```python
from build123d import *

# Parameters (mm, degrees)
BOSS_EXTRUDE1_DEPTH      = 5
BOSS_EXTRUDE1_DEPTH_BACK = 5
BODY_MOVE_COPY1_ANGLE    = 90
CUT_EXTRUDE2_DEPTH       = 708.325596879
CUT_EXTRUDE2_DEPTH_BACK  = 708.325596879
CUT_EXTRUDE3_DEPTH       = 30.3


with BuildPart() as part:
    # Sketch1 → Boss-Extrude1 (new, two sides: drawn at the far end of the back side and taken through both)
    with BuildSketch(Plane(origin=(164.5, 164.5, 0), x_dir=(-0.7071067811865478, 0.7071067811865475, 0), z_dir=(-0.7071067811865475, -0.7071067811865478, 0)).offset(-BOSS_EXTRUDE1_DEPTH_BACK)):
        Polygon((182.63813101, -115), (282.63813101, -115), (692.914393031, 0), (692.914393031, 10), (-227.63813101, 10), (-227.63813101, 0), align=None)
    extrude(amount=BOSS_EXTRUDE1_DEPTH + BOSS_EXTRUDE1_DEPTH_BACK)


with BuildPart() as part_1:
    # Body-Move/Copy1: moved
    add(part.part.moved(Location((0, 0, 0))).rotate(Axis((0, 329, 0), (0, 0, -1)), BODY_MOVE_COPY1_ANGLE))

    # Sketch2 → Cut-Extrude2 (cut, two sides: drawn at the far end of the back side and taken through both)
    with BuildSketch(Plane(origin=(-164.5, 164.5, 0), x_dir=(0.6804138174397739, 0.6804138174397697, 0.27216552697590835), z_dir=(-0.7071067811865454, 0.7071067811865498, 0)).offset(-CUT_EXTRUDE2_DEPTH_BACK)):
        Polygon((216.03456329, 71.496106715), (226.234418046, 74.381061301), (243.470750707, 13.992557954), (232.982220817, 11.02595371), align=None)
    extrude(amount=CUT_EXTRUDE2_DEPTH + CUT_EXTRUDE2_DEPTH_BACK, mode=Mode.SUBTRACT)

    # Sketch3 → Cut-Extrude3 (cut)
    with BuildSketch(Plane.XY.offset(115)):
        Polygon((-24.960869376, 311.110198436), (-17.889801564, 304.039130624), (-10.394469683, 311.534462505), (-17.465537495, 318.605530317), align=None)
        Polygon((10.394469683, 346.465537495), (17.465537495, 339.394469683), (24.960869376, 346.889801564), (17.889801564, 353.960869376), align=None)
    extrude(amount=-CUT_EXTRUDE3_DEPTH, mode=Mode.SUBTRACT)


solid = part_1.part
```
Build history of the part. All positions in model axes, mm. A direction names the side the tool comes from. Round coordinates to 2 decimals unless told otherwise and drop trailing zeros. Loops run counter-clockwise (first coordinate to the right, second up) from the corner with the lowest first, then second, coordinate; pieces in that order, holes last.
Item 1: Drill centre lines: line 1 along Y through (x, z) = (-17, 27.5); line 2 along X through (y, z) = (261, 7); line 3 along X through (y, z) = (366.5, 87). Where is each one in solid material? Low to high.
Item 2: Saw through at D-D (x = -52). List the corners of the cut face in (y, z), then the cut area to 3 significant figures.
Item 3: Saw through at C-C (y = 264). List the corners of the cut face in (x, z).
Item 4: Saw through at B-B (z = 102). List the corners of the cut face in (x, y), then the cut area to 3 significant figures.
Item 5: Which spindle directions (+Z, -Z, +X, -X, +Y, -Y) get a long thin tool onto all of the face, cutting with end or side? Do faces 1 (the face through (18, 347, 84.7)), 2 (the face through (167, 496, -10)). Say none if no direction does.
Item 6: Saw through at A-A (z = 20). List the corners of the cut face in (x, y).
Item 7: Pin check, flat tips, straight feed: P1, Ø2, axis at x = 113.5, z = 19, coming from the -Y side; P2, Ø16, axis at x = -17.5, y = 312, coming from the +Z side; P3, Ø10, axis at x = 108.5, y = 431, coming from the +Z side; P4, Ø1.5, axis at x = -69.5, z = 29.5, coming from the +Y side. Stop position of each tip, or through.
Worked answers:
1. line 1: y = 304.93 to 319.07
1. line 2: x = -75.07 to -60.93
1. line 3: x = 30.43 to 44.57
2. outline: (269.93, -10) - (284.07, -10) - (284.07, 109.8) - (269.93, 107) - close
2. area: 1,670 mm2
3. outline: (-72.07, -10) - (-57.93, -10) - (-57.93, 104.65) - (-72.07, 101.85) - close
4. outline: (-71.69, 264.39) - (-64.61, 257.31) - (-17.89, 304.04) - (-24.96, 311.11) - close; (-17.47, 318.61) - (-10.39, 311.53) - (17.47, 339.39) - (10.39, 346.47) - close; (17.89, 353.96) - (24.96, 346.89) - (71.69, 393.61) - (64.61, 400.69) - close
4. area: 1,720 mm2
5. face 1: +Z
5. face 2: -Z, +X, -X, +Y, -Y
6. outline: (-278.55, 57.52) - (-271.48, 50.45) - (-0.26, 321.67) - (-7.33, 328.74) - close; (0.26, 336.33) - (7.33, 329.26) - (278.55, 600.48) - (271.48, 607.55) - close
7. P1: stops at y = 434.43
7. P2: stops at z = 115
7. P3: stops at z = 88.7
7. P4: stops at y = 267.32
